from build123d import *

# Parameters (mm, degrees)
SKETCH1_W           = 54.5
SKETCH1_H           = 44
BOSS_EXTRUDE1_DEPTH = 42
CHAMFER2_SIZE       = 14
CHAMFER3_SIZE       = 10
CHAMFER3_SIZE_2     = 7.071067812
BOSS_EXTRUDE2_DEPTH = 6
SKETCH4_W           = 20
SKETCH4_H           = 44
SKETCH4_R           = 1.5
BOSS_EXTRUDE3_DEPTH = 4
SKETCH5_W           = 21
SKETCH5_H           = 30
CUT_EXTRUDE1_DEPTH  = 12
SKETCH6_W           = 12
SKETCH6_H           = 42
CUT_EXTRUDE2_DEPTH  = 2


with BuildPart() as part:
    # Sketch1 → Boss-Extrude1 (new body)
    with BuildSketch(Plane(origin=(0, 0, 0), x_dir=(1, 0, 0), z_dir=(0, 1, 0))):
        Rectangle(SKETCH1_W, SKETCH1_H)
        Polygon((-6, 13), (-6, 15), (6, 15), (6, 13), (8.5, 13), (8.5, 15), (20.25, 15), (20.25, -15), (8.5, -15), (8.5, -13), (6, -13), (6, -15), (-6, -15), (-6, -13), (-8.5, -13), (-8.5, -15), (-20.25, -15), (-20.25, 15), (-8.5, 15), (-8.5, 13), align=None, mode=Mode.SUBTRACT)
    extrude(amount=BOSS_EXTRUDE1_DEPTH)

    # Chamfer2
    # the kernel refuses this chamfer: 14 mm, written as the material it takes off along each edge
    with BuildSketch(Plane(origin=(27.25, 42, 58.003561832), x_dir=(0.027495876610586365, -0.9996219169112968, 0), z_dir=(0, 0, -1)), Plane(origin=(-27.25, 42, -58.003561832), x_dir=(-0.027495876610586365, -0.9996219169112968, 0), z_dir=(0, 0, 1))) as chamfer2_piece_1:
        Polygon((CHAMFER2_SIZE * 0.999621916911, CHAMFER2_SIZE * 0.0274958766106), (-CHAMFER2_SIZE * 0.0274958766106, CHAMFER2_SIZE * 0.999621916911), (0, 0), align=None)
    extrude(amount=116.007123663, mode=Mode.SUBTRACT)

    # Chamfer3
    # the kernel refuses this chamfer: 10, 7.071067812 mm, written as the material it takes off along each edge
    with BuildSketch(Plane(origin=(20.25, 35, -15), x_dir=(0.7262819568769621, -0.6873969152643694, 0), z_dir=(0, 0, 1)), Plane(origin=(-20.25, 35, 15), x_dir=(-0.7262819568769624, -0.6873969152643691, 0), z_dir=(0, 0, -1))) as chamfer3_piece_1:
        Polygon((CHAMFER3_SIZE * 0.999621916911, -CHAMFER3_SIZE * 0.0274958766106), (CHAMFER3_SIZE_2 * 0.687396915251, -CHAMFER3_SIZE_2 * 0.726281956863), (0, 0), align=None)
    extrude(amount=30, mode=Mode.SUBTRACT)

    # Sketch2 → Boss-Extrude2 (add)
    with BuildSketch(Plane.XY.offset(-15)):
        Polygon((-27.25, 20.928932188), (-6.178932188, 42), (-13.25, 42), (-27.25, 28), align=None)
        Polygon((13.25, 42), (6.178932188, 42), (27.25, 20.928932188), (27.25, 28), align=None)
    boss_extrude2 = extrude(amount=BOSS_EXTRUDE2_DEPTH)

    # Mirror2: Boss-Extrude2 across plane
    add(boss_extrude2.mirror(Plane.XY))

    # Sketch4 → Boss-Extrude3 (add)
    # profile 1 of 2: a face of its own
    with BuildSketch(Plane.XZ):
        with Locations((37.25, 0)):
            Rectangle(SKETCH4_W, SKETCH4_H)
        with Locations(Location((40.25, 15, 0), (0, 0, 270))):
            Circle(SKETCH4_R, mode=Mode.SUBTRACT)
        with Locations(Location((40.25, -15, 0), (0, 0, 90))):
            Circle(SKETCH4_R, mode=Mode.SUBTRACT)
    # profile 2 of 2: a face of its own
    with BuildSketch(Plane.XZ):
        with Locations((-37.25, 0)):
            Rectangle(SKETCH4_W, SKETCH4_H)
        with Locations(Location((-40.25, -15, 0), (0, 0, 270))):
            Circle(SKETCH4_R, mode=Mode.SUBTRACT)
        with Locations(Location((-40.25, 15, 0), (0, 0, 90))):
            Circle(SKETCH4_R, mode=Mode.SUBTRACT)
    extrude(amount=-BOSS_EXTRUDE3_DEPTH)

    # Sketch5 → Cut-Extrude1 (cut)
    with BuildSketch(Plane(origin=(0, 42, 0), x_dir=(1, 0, 0), z_dir=(0, 1, 0))):
        Rectangle(SKETCH5_W, SKETCH5_H)
    extrude(amount=-CUT_EXTRUDE1_DEPTH, mode=Mode.SUBTRACT)

    # Sketch6 → Cut-Extrude2 (cut)
    with BuildSketch(Plane(origin=(0, 0, 15), x_dir=(-1, 0, 0), z_dir=(0, 0, -1))):
        with Locations((0, 21)):
            Rectangle(SKETCH6_W, SKETCH6_H)
    cut_extrude2 = extrude(amount=-CUT_EXTRUDE2_DEPTH, mode=Mode.SUBTRACT)

    # Mirror3: Cut-Extrude2 across plane
    add(cut_extrude2.mirror(Plane.XY), mode=Mode.SUBTRACT)


solid = part.part
Geometry check sheet. Reference: the model listing, model coordinates, mm. A direction names the side the tool comes from. Coordinates: 2 decimals unless noted, no trailing zeros. Order: outer loops, then holes, each group sorted by start corner. A loop starts at its lowest first (then second) coordinate and runs counter-clockwise, first axis right, second up. Notation, with made-up numbers: (-15, 5.5) -> (-10, 5.5) arc R16 cw to (-10, 18.5) -> close; hole circle Ø5 at (16.25, -32). An arc over 180 degrees is marked (long way). Use a Markdown table: item, result. Add a question column.
1. Cross-section at D-D (y = 27). Enter the section's corners in (x, z).
2. Material ranges on L1, parallel to X at y = 15, z = 14; L2, parallel to Z at x = -8.5, y = 31.5; L3, parallel to X at y = 11, z = -16, recorded low to high.
3. Cross-section at A-A (x = -40.25). Enter the section's corners in (y, z).
4. Go/stop test with flat-tipped pins: pin 1 Ø19 at (y, z) = (15, -8.5) entering from -X; pin 2 Ø4.5 at (y, z) = (16.5, -15.5) entering from +X; pin 3 Ø1.3 at (y, z) = (39.5, -11.5) entering from -X. Record where each tip stops, or that it passes through.
5. Set-up check for faces 1 (the face through (-6, 16, 15)), 2 (the face through (27.25, 16, 0)), 3 (the face through (-15.44, 32.74, 12.04)), 4 (the face through (7, 30, 14)), 5 (the face through (-27.25, 16, 0)): record each of +Z, -Z, +X, -X, +Y, -Y from which the full face is reachable in a straight line by a thin tool's end or side.
6. Cross-section at C-C (y = 39). Enter the section's corners in (x, z), and give its area (3 significant figures).
7. Mould release check, pull along Z, two halves, no side actions. Record for faces 6 (the face through (0, 21, 17)), 7 (the face through (-37, 4, 0)), 8 (the face through (-1, 16, 22)): pulls with the +Z half, pulls with the -Z half, needs draft (parallel to the pull), parting line crosses it, or undercut.
8. Cross-section at B-B (z = 2). Enter the section's corners in (x, y), and give its area (3 significant figures).
Filled sheet:
| question | item | result |
|---|---|---|
| 1 | outline | (-27.25, -22) -> (27.25, -22) -> (27.25, 22) -> (-27.25, 22) -> close; hole (-20.25, -15) -> (-8.5, -15) -> (-8.5, -13) -> (-6, -13) -> (-6, -17) -> (6, -17) -> (6, -13) -> (8.5, -13) -> (8.5, -15) -> (20.25, -15) -> (20.25, 15) -> (8.5, 15) -> (8.5, 13) -> (6, 13) -> (6, 17) -> (-6, 17) -> (-6, 13) -> (-8.5, 13) -> (-8.5, 15) -> (-20.25, 15) -> close |
| 2 | L1 | -27.25 to -20.25, -8.5 to -6, 6 to 8.5, 20.25 to 27.25 |
| 2 | L2 | -22 to -15, 15 to 22 |
| 2 | L3 | -27.25 to -6, 6 to 27.25 |
| 3 | outline | (0, -22) -> (4, -22) -> (4, -16.5) -> (0, -16.5) -> close; (0, -13.5) -> (4, -13.5) -> (4, 13.5) -> (0, 13.5) -> close; (0, 16.5) -> (4, 16.5) -> (4, 22) -> (0, 22) -> close |
| 4 | pin 1 | x = -27.25 |
| 4 | pin 2 | x = 27.25 |
| 4 | pin 3 | x = -16.4 |
| 5 | face 1 | +Y, -Y |
| 5 | face 2 | +Z, -Z, +X, +Y |
| 5 | face 3 | -Y |
| 5 | face 4 | +Y |
| 5 | face 5 | +Z, -Z, -X, +Y |
| 6 | outline | (-16.25, -22) -> (16.25, -22) -> (16.25, -9) -> (10.5, -9) -> (10.5, -15) -> (6, -15) -> (6, -17) -> (-6, -17) -> (-6, -15) -> (-10.5, -15) -> (-10.5, -9) -> (-16.25, -9) -> close; (-16.25, 9) -> (-10.5, 9) -> (-10.5, 15) -> (-6, 15) -> (-6, 17) -> (6, 17) -> (6, 15) -> (10.5, 15) -> (10.5, 9) -> (16.25, 9) -> (16.25, 22) -> (-16.25, 22) -> close |
| 6 | area | 545 mm2 |
| 7 | face 6 | undercut |
| 7 | face 7 | needs draft |
| 7 | face 8 | pulls with the +Z half |
| 8 | outline | (-47.25, 0) -> (-20.25, 0) -> (-20.25, 27.93) -> (-27.25, 27.93) -> (-27.25, 4) -> (-47.25, 4) -> close; (20.25, 0) -> (47.25, 0) -> (47.25, 4) -> (27.25, 4) -> (27.25, 27.93) -> (20.25, 27.93) -> close |
| 8 | area | 551 mm2 |
